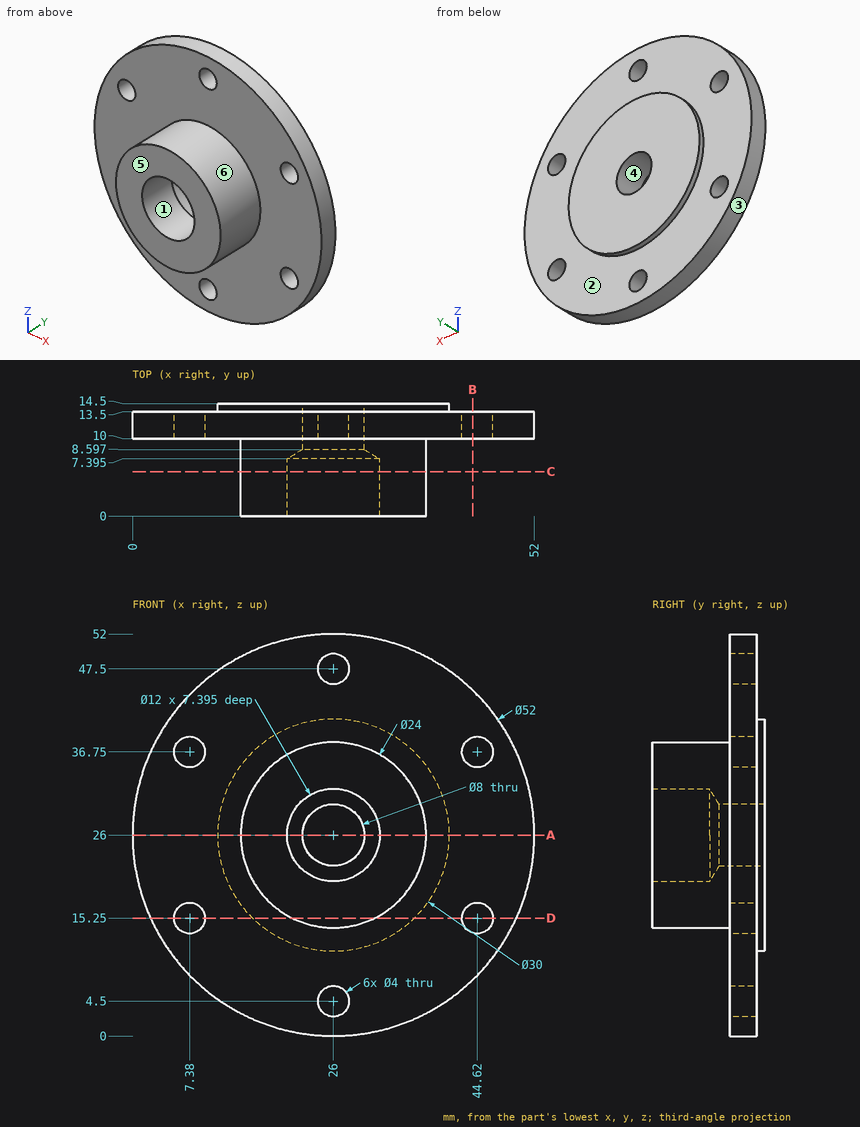
Part print with two shaded views. Sizes in mm from the minimum x, y, z corner. A direction names the side the tool comes from. Coordinates: 2 decimals unless noted, no trailing zeros. Loops run counter-clockwise (first coordinate to the right, second up) from the corner with the lowest first, then second, coordinate; pieces in that order, holes last. Notation, with made-up numbers: M 77.25,-4.5 L 93.25,-4.5 A15 cw 93.25,16.5 Z; hole C 32.25,22.25 d11. An arc over 180 degrees is marked long. Use CSV: the item, a comma, the result in double quotes. Start each with the question number.
1. Flat gauge pins, fed straight in: pin 1 (3.5 mm diameter, centred on x = 26, z = 47.5, fed in from +Y); pin 2 (3 mm diameter, centred on x = 21.5, y = 7, fed in from -Z); pin 3 (19 mm diameter, centred on x = 26, z = 26, fed in from -Y); pin 4 (4 mm diameter, centred on x = 35, y = 5, fed in from -Z). Where does each tip first touch, or does it go through?
2. Band-saw the part on B-B, the plane x = 44. List the corners of the cut face in (y, z), then the cut area to 3 significant figures.
3. Band-saw the part on C-C, the plane y = 5.75. List the corners of the cut face in (x, z).
4. Band-saw the part on A-A, the plane z = 26. List the corners of the cut face in (x, y) (1 decimal).
5. Band-saw the part on D-D, the plane z = 15.25. List the corners of the cut face in (x, y).
6. Probe probe 1 along X at (y, z) = (11.1, 15.25) (1 decimal); probe 2 along Z at (x, y) = (26, 5); probe 3 along Y at (x, z) = (33, 5.5). List the from-to ranges inside material, lowest first. Write a range as [from, to].
7. Tool access for the marked faces 1, 2 and 3: list every direction of +Z, -Z, +X, -X, +Y, -Y with a clear straight run to the whole face (end or side of a thin tool).
8. Two-plate mould, pull along X, no slides. Class the marked faces 4, 5 and 6: pulls with the +X half, pulls with the -X half, needs draft (parallel to the pull), parting line crosses it, or undercut.
Entries:
1,pin 1,"passes through"
1,pin 2,"stops at z = 14.38"
1,pin 3,"stops at y = 0"
1,pin 4,"stops at z = 16.25"
2,outline,"M 10,7.24 L 13.5,7.24 L 13.5,13.35 L 10,13.35 Z; M 10,17.15 L 13.5,17.15 L 13.5,34.85 L 10,34.85 Z; M 10,38.65 L 13.5,38.65 L 13.5,44.76 L 10,44.76 Z"
2,area,"105 mm2"
3,outline,"C 26,26 d24; hole C 26,26 d12"
4,outline,"M 0,10 L 14,10 L 14,0 L 20,0 L 20,7.4 L 22,8.6 L 22,14.5 L 11,14.5 L 11,13.5 L 0,13.5 Z; M 30,8.6 L 32,7.4 L 32,0 L 38,0 L 38,10 L 52,10 L 52,13.5 L 41,13.5 L 41,14.5 L 30,14.5 Z"
5,outline,"M 2.33,10 L 5.38,10 L 5.38,13.5 L 2.33,13.5 Z; M 9.38,10 L 20.67,10 L 20.67,0 L 31.33,0 L 31.33,10 L 42.62,10 L 42.62,13.5 L 36.46,13.5 L 36.46,14.5 L 15.54,14.5 L 15.54,13.5 L 9.38,13.5 Z; M 46.62,10 L 49.67,10 L 49.67,13.5 L 46.62,13.5 Z"
6,probe 1,"x = [2.3, 5.4], [9.4, 42.6], [46.6, 49.7]"
6,probe 2,"z = [14, 20], [32, 38]"
6,probe 3,"y = [10, 13.5]"
7,face 1,"-Y"
7,face 2,"+Y"
7,face 3,"+Y, -Y"
8,face 4,"undercut"
8,face 5,"needs draft"
8,face 6,"parting line crosses it"
